The model under review builds one solid part; all positions refer to its coordinate system, in mm. Face numbers are marked on the shaded views. A direction names the side the tool comes from. Coordinates: 2 decimals unless noted, no trailing zeros. Loops run counter-clockwise (first coordinate to the right, second up) from the corner with the lowest first, then second, coordinate; pieces in that order, holes last. Notation, with made-up numbers: (-27.5, 17.5) - (-19.5, 17.5) arc R23 cw to (-19.5, 27.5) - close; hole circle Ø4 at (-15, 33.25). An arc over 180 degrees is marked (long way). One line per item, written item: value. Start each with the question number.
1. Insertion check: P1, Ø2, axis at x = 15, z = 19.5, coming from the +Y side; P2, Ø5, axis at y = 9.15, z = 40.5, coming from the +X side. Each pin has a flat end and moves straight along its axis. Give the tip position at first contact, or say it passes through.
2. We need section D-D, the plane y = 34. Give the boundary of the cut face in (x, z).
3. Mouldability with a two-part tool opening along Z and no side actions: class the marked faces 3, 4 and 5 as +Z half, -Z half, draft (parallel to the pull), parting line (faces both ways), or undercut.
4. To check wall thickness, follow line 1 (Z direction, x = -1, y = 9); line 2 (Z direction, x = 5, y = -1); line 3 (Y direction, x = -1, z = 40). State the ranges of each line that lie inside material, in increasing order.
5. For the marked faces 1 and 2, list the 3-axis set-ups (+Z, -Z, +X, -X, +Y, -Y) from which the entire face can be reached by the end or side of a thin tool; tool diameter is ignored.
6. We need section A-A, the plane y = 40.15. Give the boundary of the cut face in (x, z).
7. We need section B-B, the plane z = 25. Give the boundary of the cut face in (x, y), then the cut area to 3 significant figures.
8. We need section C-C, the plane x = 21. Give the boundary of the cut face in (y, z).
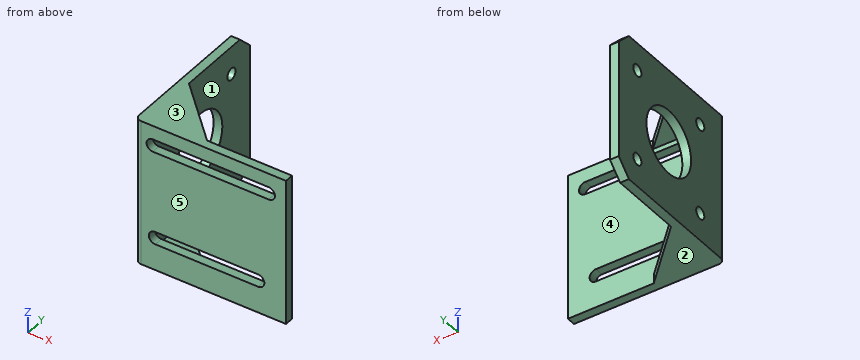
from build123d import *

# Parameters (mm, degrees)
BOSS_EXTRUDE1_DEPTH = 50
RIB1_REACH          = 87.339
SKETCH8_WALL_W      = 200.043796972
SKETCH8_WALL_H      = 3
RIB2_REACH          = 87.339
SKETCH10_WALL_W     = 199.830842734
SKETCH10_WALL_H     = 3
FILLET1_R           = 2
SKETCH11_R          = 11
SKETCH11_R_2        = 2
CUT_EXTRUDE1_DEPTH  = 50
CHAMFER1_SIZE       = 5
CUT_EXTRUDE2_DEPTH  = 50


with BuildPart() as part:
    # Sketch1 → Boss-Extrude1 (new body)
    with BuildSketch(Plane.XY):
        Polygon((0, 0), (0, 49.3), (-3, 49.3), (-3, -3), (48.5, -3), (48.5, 0), align=None)
    extrude(amount=BOSS_EXTRUDE1_DEPTH)

    # Sketch8 wall → Rib1 (add, up to next)
    with BuildSketch(Plane(origin=(9.75, 9.6, 50), x_dir=(0.712566819448, -0.701604252995, 0), z_dir=(0.701604252995, 0.712566819448, 0)), mode=Mode.PRIVATE) as rib1_sk1:
        with Locations((0, 1.5)):
            Rectangle(SKETCH8_WALL_W, SKETCH8_WALL_H)
    rib1_tool1 = extrude(rib1_sk1.sketch, amount=-RIB1_REACH, mode=Mode.PRIVATE) - part.part
    add(rib1_tool1.solids().sort_by_distance((9.75, 9.6, 50))[0])

    # Sketch10 wall → Rib2 (add, up to next)
    with BuildSketch(Plane(origin=(9.6, 9.6, 0), x_dir=(0.707106781187, -0.707106781187, 0), z_dir=(0.707106781187, 0.707106781187, 0)), mode=Mode.PRIVATE) as rib2_sk1:
        with Locations((0, -1.5)):
            Rectangle(SKETCH10_WALL_W, SKETCH10_WALL_H)
    rib2_tool1 = extrude(rib2_sk1.sketch, amount=-RIB2_REACH, mode=Mode.PRIVATE) - part.part
    add(rib2_tool1.solids().sort_by_distance((9.6, 9.6, 0))[0])

    # Fillet1
    fillet1_edges = [part.edges().sort_by_distance(p)[0] for p in [
        (-3, -3, 25),
    ]]
    fillet(fillet1_edges, radius=FILLET1_R)

    # Sketch11 → Cut-Extrude1 (cut)
    with BuildSketch(Plane(origin=(0, 0, 0), x_dir=(0, 0, -1), z_dir=(1, 0, 0))):
        with Locations(Location((-25, 24.65, 0), (0, 0, 90))):
            Circle(SKETCH11_R)
        with Locations(Location((-40.5, 40.15, 0), (0, 0, 90))):
            Circle(SKETCH11_R_2)
        with Locations(Location((-9.5, 40.15, 0), (0, 0, 90))):
            Circle(SKETCH11_R_2)
        with Locations(Location((-9.5, 9.15, 0), (0, 0, 90))):
            Circle(SKETCH11_R_2)
        with Locations(Location((-40.5, 9.15, 0), (0, 0, 90))):
            Circle(SKETCH11_R_2)
    extrude(amount=-CUT_EXTRUDE1_DEPTH, mode=Mode.SUBTRACT)

    # Chamfer1
    chamfer1_edges = [part.edges().sort_by_distance(p)[0] for p in [
        (-1.5, 49.3, 50),
        (-1.5, 49.3, 0),
    ]]
    chamfer(chamfer1_edges, length=CHAMFER1_SIZE)

    # Sketch12 → Cut-Extrude2 (cut)
    with BuildSketch(Plane.XZ.offset(3)):
        with BuildLine():
            Line((38.94922721, 9), (3.928025493, 9))
            ThreePointArc((3.928025493, 9), (1.678310919, 11.099272288), (3.828882318, 13.3))
            Line((3.828882318, 13.3), (38.94922721, 13.3))
            ThreePointArc((38.94922721, 13.3), (41.09922721, 11.15), (38.94922721, 9))
        make_face()
        with BuildLine():
            Line((3.039672714, 41), (42.571371384, 41))
            ThreePointArc((42.571371384, 41), (44.721371384, 43.15), (42.571371384, 45.3))
            Line((42.571371384, 45.3), (3.039672714, 45.3))
            ThreePointArc((3.039672714, 45.3), (0.889672714, 43.15), (3.039672714, 41))
        make_face()
    extrude(amount=-CUT_EXTRUDE2_DEPTH, mode=Mode.SUBTRACT)


solid = part.part
Findings below:
1. P1: y = 0
1. P2: x = 0
2. outline: (-3, 0) - (0, 0) - (0, 19.21) - (-3, 19.21) - close; (-3, 30.79) - (0, 30.79) - (0, 50) - (-3, 50) - close
3. face 3: +Z half
3. face 4: undercut
3. face 5: draft
4. line 1: 0 to 7.51, 11.49 to 38.51, 42.49 to 50
4. line 2: 0 to 9, 13.3 to 41, 45.3 to 50
4. line 3: -3 to 7.21, 11.09 to 38.21, 42.09 to 49.3
5. face 1: +X, +Y
5. face 2: -Z, +X, -X, +Y, -Y
6. outline: (-3, 0) - (0, 0) - (0, 7.5) - (-3, 7.5) - close; (-3, 11.5) - (0, 11.5) - (0, 38.5) - (-3, 38.5) - close; (-3, 42.5) - (0, 42.5) - (0, 50) - (-3, 50) - close
7. outline: (-3, -1) arc R2 ccw to (-1, -3) - (48.5, -3) - (48.5, 0) - (0, 0) - (0, 13.65) - (-3, 13.65) - close; (-3, 35.65) - (0, 35.65) - (0, 49.3) - (-3, 49.3) - close
7. area: 236 mm2
8. outline: (-3, 0) - (0, 0) - (0, 9) - (-3, 9) - close; (-3, 13.3) - (0, 13.3) - (0, 41) - (-3, 41) - close; (-3, 45.3) - (0, 45.3) - (0, 50) - (-3, 50) - close
